CAD build for the part. Positions are in the model's coordinates, mm. Face numbers are marked on the shaded views. A direction names the side the tool comes from. Give positions to 0.01 mm unless a question says otherwise; leave off trailing zeros. Order: outer loops, then holes, each group sorted by start corner. A loop starts at its lowest first (then second) coordinate and runs counter-clockwise, first axis right, second up. Notation, with made-up numbers: M -34.5,-39.5 L 23.5,-39.5 A24 cw 23.5,-26.5 Z; hole C 29.5,-24.5 d4. An arc over 180 degrees is marked long. Put each result on its own line as item: value. Start each with the question number.
1) Cut at B-B (y = 6.5). Write the cut outline in (x, z).
2) Tool access for the marked faces 4, 5, 6 and 7: list every direction of +Z, -Z, +X, -X, +Y, -Y with a clear straight run to the whole face (end or side of a thin tool).
3) Cut at D-D (x = -55). Write the cut outline in (y, z), and give its area (3 significant figures).
4) Pin check, flat tips, straight feed: pin 1 (1.9 mm diameter, centred on x = -18, y = -8, fed in from -Z); pin 2 (22 mm diameter, centred on x = -17, y = -0.5, fed in from +Z); pin 3 (1 mm diameter, centred on x = 18, z = -4, fed in from -Y). Stop position of each tip, or through.
5) Two-plate mould, pull along Z, no slides. Class the marked faces 1, 2 and 3: released by +Z, released by -Z, zero draft, split by the parting line, or undercut.
6) Cut at C-C (y = 0). Write the cut outline in (x, z).
7) Drill centre lines: line 1 (X direction, y = -5, z = -7.5); line 2 (Z direction, x = -5.5, y = -8); line 3 (Z direction, x = 55, y = -7). Where is each one in solid material? Low to high. Write a range as [from, to].
8) Cut at A-A (x = 55). Write the cut outline in (y, z).
```python
from build123d import *

# Parameters (mm, degrees)
SKETCH2_R           = 10
SKETCH2_R_2         = 6
BOSS_EXTRUDE1_DEPTH = 21.5
BOSS_EXTRUDE2_DEPTH = 10
CUT_EXTRUDE1_DEPTH  = 6.25
FILLET1_R           = 20
FILLET2_R           = 2.5
MOVE_FACE1_BY       = 9
MOVE_FACE2_BY       = 9
MOVE_FACE3_BY       = 2


with BuildPart() as part:
    # Sketch2 → Boss-Extrude1 (new, symmetric)
    with BuildSketch(Plane(origin=(0, 0, 0), x_dir=(1, 0, 0), z_dir=(0, 1, 0))):
        with Locations(Location((-55, 7.5, 0), (0, 0, 270))):
            Circle(SKETCH2_R)
        with Locations(Location((-55, 7.5, 0), (0, 0, 270))):
            Circle(SKETCH2_R_2, mode=Mode.SUBTRACT)
    extrude(amount=BOSS_EXTRUDE1_DEPTH, both=True)

    # Sketch2<3> → Boss-Extrude2 (add, symmetric)
    with BuildSketch(Plane(origin=(0, 0, 0), x_dir=(1, 0, 0), z_dir=(0, 1, 0))):
        with BuildLine():
            Line((0, 0), (0, 7.5))
            Line((0, 7.5), (-45, 7.5))
            ThreePointArc((-45, 7.5), (-45.885621722, 3.385621722), (-48.385621722, 0))
            Line((-48.385621722, 0), (0, 0))
        make_face()
        with BuildLine():
            Line((-45, 7.5), (0, 7.5))
            Line((0, 7.5), (0, 15))
            Line((0, 15), (-48.385621722, 15))
            ThreePointArc((-48.385621722, 15), (-45.885621722, 11.614378278), (-45, 7.5))
        make_face()
    extrude(amount=BOSS_EXTRUDE2_DEPTH, both=True)

    # Mirror1: part across plane


with BuildPart() as part_1:
    add(part.part)
    add(part.part.mirror(Plane(origin=(0, 10, 0), x_dir=(0, 0, 1), z_dir=(-1, 0, 0))))

    # Sketch3 → Cut-Extrude1 (cut)
    with BuildSketch(Plane(origin=(0, 10, 0), x_dir=(1, 0, 0), z_dir=(0, 1, 0))):
        with BuildLine():
            Line((40.813739041, 10.5), (-40.813739041, 10.5))
            ThreePointArc((-40.813739041, 10.5), (-40.5, 7.5), (-40.813739041, 4.5))
            Line((-40.813739041, 4.5), (40.813739041, 4.5))
            ThreePointArc((40.813739041, 4.5), (40.5, 7.5), (40.813739041, 10.5))
        make_face()
    cut_extrude1 = extrude(amount=-CUT_EXTRUDE1_DEPTH, mode=Mode.SUBTRACT)

    # Mirror2: Cut-Extrude1 across plane
    add(cut_extrude1.mirror(Plane.ZX), mode=Mode.SUBTRACT)

    # Fillet1
    fillet1_edges = [part_1.edges().sort_by_distance(p)[0] for p in [
        (-48.385621722, 0, -15),
        (-48.385621722, 0, 0),
        (48.385621722, 0, 0),
        (48.385621722, 0, -15),
    ]]
    fillet(fillet1_edges, radius=FILLET1_R)

    # Fillet2
    fillet2_edges = [part_1.edges().sort_by_distance(p)[0] for p in [
        (-40.813739041, 6.875, -4.5),
        (-40.813739041, 6.875, -10.5),
        (40.813739041, 6.875, -10.5),
        (40.813739041, 6.875, -4.5),
        (-40.813739041, -6.875, -10.5),
        (-40.813739041, -6.875, -4.5),
        (40.813739041, -6.875, -4.5),
        (40.813739041, -6.875, -10.5),
    ]]
    fillet(fillet2_edges, radius=FILLET2_R)

    # Move Face1: a face moved inward by 9.0
    extrude(part_1.faces().sort_by_distance((-55, 21.5, 0.5))[0], amount=MOVE_FACE1_BY, dir=(0, -1, 0), mode=Mode.SUBTRACT)

    # Move Face2: a face moved inward by 9.0
    extrude(part_1.faces().sort_by_distance((-55, -21.5, 0.5))[0], amount=MOVE_FACE2_BY, dir=(0, 1, 0), mode=Mode.SUBTRACT)

    # Move Face3: a curved face moved outward by 2.0
    add(Solid.thicken(part_1.faces().sort_by_distance((-55, 0, -13.5))[0], MOVE_FACE3_BY))


solid = part_1.part
```
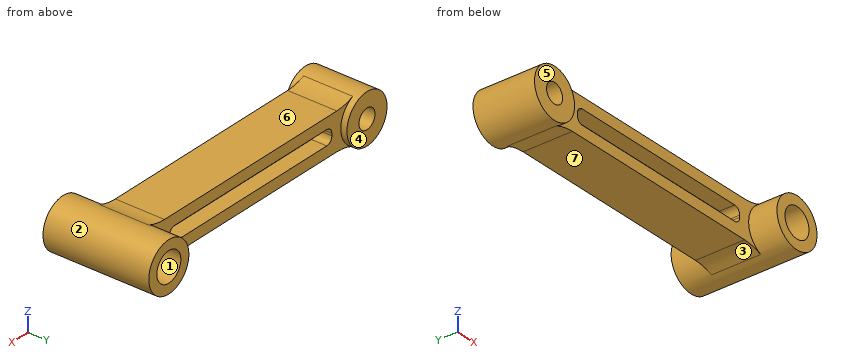
Solution:
1. outline: M -51,-16.67 A20 cw -43.01,-15 L 43.01,-15 A20 cw 51,-16.67 A10 ccw long 51,1.67 A20 cw 43.01,0 L -43.01,0 A20 cw -51,1.67 A10 ccw long Z; hole C -55,-7.5 d8; hole M -40.51,-7.93 A2.5 ccw -38.01,-10.5 L 38.01,-10.5 A2.5 ccw 40.51,-7.93 A14.5 cw 40.51,-7.07 A2.5 ccw 38.01,-4.5 L -38.01,-4.5 A2.5 ccw -40.51,-7.07 A14.5 cw Z; hole C 55,-7.5 d12
2. face 4: +Z, -Z, -X, +Y
2. face 5: +Z, -Z, -X, -Y
2. face 6: +Z, +Y, -Y
2. face 7: -Z, +Y, -Y
3. outline: M -12.5,-17.5 L 12.5,-17.5 L 12.5,-11.5 L -12.5,-11.5 Z; M -12.5,-3.5 L 12.5,-3.5 L 12.5,2.5 L -12.5,2.5 Z
3. area: 300 mm²
4. pin 1: z = -15
4. pin 2: z = 0
4. pin 3: y = -10
5. face 1: undercut
5. face 2: split by the parting line
5. face 3: released by -Z
6. outline: M -51,-16.67 A20 cw -43.01,-15 L 43.01,-15 A20 cw 51,-16.67 A10 ccw long 51,1.67 A20 cw 43.01,0 L -43.01,0 A20 cw -51,1.67 A10 ccw long Z; hole C -55,-7.5 d8; hole C 55,-7.5 d12
7. line 1: [-65, -59], [-51, -40.5], [40.5, 49], [61, 65]
7. line 2: [-15, -10.5], [-4.5, 0]
7. line 3: [-17.5, -13.5], [-1.5, 2.5]
8. outline: M -21.5,-17.5 L 21.5,-17.5 L 21.5,-13.5 L -21.5,-13.5 Z; M -21.5,-1.5 L 21.5,-1.5 L 21.5,2.5 L -21.5,2.5 Z
